Autodesk Inventor part; units mm, degrees
ref_plane "YZ Plane" through (0, 0, 0) normal (1, 0, 0) x (0, 1, 0)
ref_plane "XZ Plane" through (0, 0, 0) normal (0, 1, 0) x (-1, 0, 0)
ref_plane "XY Plane" through (0, 0, 0) normal (0, 0, 1) x (1, 0, 0)
sketch "Sketch1" plane through (0, 0, 0) normal (0, 1, 0) x (-1, 0, 0)
  line L0 (0, 0) -> (-58.801, 0)
  line L1 (-58.801, 0) -> (-58.801, 15.875)
  line L2 (-58.801, 15.875) -> (0, 15.875)
  line L3 (0, 15.875) -> (0, 0)
  dimension "d0" = 58.801
  dimension "d1" = 15.875
extrude "Extrusion1" add sketch "Sketch1" along normal blind 5.6134
sketch "Sketch7" plane through (0, 5.6134, 0) normal (0, 1, 0) x (1, 0, 0)
  circle A0 centre (10.8966, -6.6524) radius 1.6
  circle A1 centre (47.8966, -6.6524) radius 1.6
  line L0 (0, 0) -> (0, -15.875)
  line L1 (58.801, 0) -> (0, 0)
  line L2 (58.801, -15.875) -> (58.801, 0)
  dimension "d22" = 3.2
  dimension "d23" = 3.2
  dimension "d24" = 37
  dimension "d43" = 6.6524
  dimension "d44" = 6.6524
  dimension "d48" = 10.8966
  dimension "d49" = 10.9044
extrude "Extrusion6" cut sketch "Sketch7" against normal blind 25.4
sketch "Sketch8" plane through (0, 5.6134, 0) normal (0, 1, 0) x (1, 0, 0)
  line L0 (58.801, 0) -> (0, 0)
  line L1 (0, 0) -> (0, -15.875)
  line L2 (58.801, -15.875) -> (58.801, 0)
  line L3 (0, -15.875) -> (3.175, -15.875)
  line L4 (3.175, -15.875) -> (3.175, 0)
  line L5 (3.175, 0) -> (0, 0)
  line L6 (0, 0) -> (0, -15.875)
  line L7 (58.801, -15.875) -> (55.626, -15.875)
  line L8 (55.626, -15.875) -> (55.626, 0)
  line L9 (55.626, 0) -> (58.801, 0)
  line L10 (58.801, 0) -> (58.801, -15.875)
  dimension "d34" = 3.175
  dimension "d35" = 3.175
extrude "Extrusion7" cut sketch "Sketch8" against normal blind 2.4384
equation "\"d23\" = d22"
properties part number "Lidar Sensor Case Piece 3"
Input: part model. Units: mm. Frame: model coordinates. A direction names the side the tool comes from. Round coordinates to 2 decimals unless told otherwise and drop trailing zeros. Loops run counter-clockwise (first coordinate to the right, second up) from the corner with the lowest first, then second, coordinate; pieces in that order, holes last.
1) Section query A-A on z = 14. Return the cut outline in (x, y) (3 decimals), plus the area to 3 significant figures.
Ans:
outline: (0, 0) - (58.801, 0) - (58.801, 3.175) - (55.626, 3.175) - (55.626, 5.613) - (3.175, 5.613) - (3.175, 3.175) - (0, 3.175) - close
area: 315 mm2
2) Set-up query: faces 1 (the flat face through (58.801, 2, 8)), 2 (the flat face through (57, 3.175, 8)), 3 (the flat face through (3.175, 4, 8)). Return all of +Z, -Z, +X, -X, +Y, -Y with unobstructed straight access to the full face (end or side cutting, diameter ignored); none if empty.
Ans:
face 1: +Z, -Z, +X, +Y, -Y
face 2: +Z, -Z, +X, +Y
face 3: +Z, -Z, -X, +Y
3) Section query B-B on y = 0.5. Return the cut outline in (x, z) (3 decimals), plus the area to 3 significant figures.
Ans:
outline: (0, 0) - (58.801, 0) - (58.801, 15.875) - (0, 15.875) - close; hole circle Ø3.2 at (10.897, 6.652); hole circle Ø3.2 at (47.897, 6.652)
area: 917 mm2
4) Section query C-C on y = 4. Return the cut outline in (x, z) (3 decimals), plus the area to 3 significant figures.
Ans:
outline: (3.175, 0) - (55.626, 0) - (55.626, 15.875) - (3.175, 15.875) - close; hole circle Ø3.2 at (10.897, 6.652); hole circle Ø3.2 at (47.897, 6.652)
area: 817 mm2
5) Pin query (flat end, axial travel): pin 1 (8 mm diameter, centred on x = 39, z = 10, fed in from -Y); pin 2 (0.7 mm diameter, centred on y = 4.5, z = 8, fed in from +X). Return the tip coordinate at first contact, or that it passes through.
Ans:
pin 1: stops at y = 0
pin 2: stops at x = 55.63
6) Pull-direction query (X, two-part tool) for faces 4 (the flat face through (0, 2, 8)), 5 (the flat face through (55.626, 4, 8)), 6 (the cylindrical face through (12.375, 2.846, 7.265)), 7 (the flat face through (2, 3.175, 8)); classes: released by +X, released by -X, zero draft, split by the parting line, or undercut.
Ans:
face 4: released by -X
face 5: released by +X
face 6: undercut
face 7: zero draft
7) Material intervals for line 1 (X direction, y = 1.9, z = 5.5); line 2 (Z direction, x = 11, y = 4.1) (3 decimals); line 3 (X direction, y = 4, z = 15.25) (3 decimals), sorted ascending.
Ans:
line 1: x = 0 to 9.79, 12.01 to 46.79, 49.01 to 58.8
line 2: z = 0 to 5.056, 8.249 to 15.875
line 3: x = 3.175 to 55.626
